Design review of the part built by this model. Coordinates are the model's own, in mm. A direction names the side the tool comes from. Round coordinates to 2 decimals unless told otherwise and drop trailing zeros. Loops run counter-clockwise (first coordinate to the right, second up) from the corner with the lowest first, then second, coordinate; pieces in that order, holes last. Notation, with made-up numbers: (24.5, -16) - (74.5, -16) arc R12 cw to (74.5, -1) - close; hole circle Ø3 at (-23.5, 29.5). An arc over 180 degrees is marked (long way). Return JSON: item names as keys, results as strings. Group by question number.
(1) For faces 1 (the flat face through (-35, 14, -54)), 2 (the cylindrical face through (-37.028, 16.354, -4.888)), 3 (the flat face through (-39, 13, -54)), list the 3-axis set-ups (+Z, -Z, +X, -X, +Y, -Y) from which the entire face can be reached by the end or side of a thin tool; tool diameter is ignored.
(2) The part is to be moulded in two halves that separate along X. For faces 4 (the cylindrical face through (-37.03, 17.69, -51.32)), 5 (the cylindrical face through (-42.33, 1.97, -51.95)), 6 (the flat face through (-35, 14, -5)), say which applies: pulls with the +X half, pulls with the -X half, needs draft (parallel to the pull), parting line crosses it, or undercut.
(3) We need section A-A, the plane x = -36.5. Write out the cut boundary in (y, z), and give its area (3 significant figures).
(4) Clearance check with flat-ended pins moving along their axes: pin 1 (4 mm diameter, centred on x = -32.5, z = -21.5, fed in from +Y); pin 2 (3 mm diameter, centred on x = -37, z = -51.5, fed in from +Y); pin 3 (2.5 mm diameter, centred on y = 14, z = -55, fed in from -X). State where each tip first meets the part, or that it passes through.
(5) We need section C-C, the plane z = -18.45. Write out the cut boundary in (x, y).
(6) We need section D-D, the plane z = -53.4. Write out the cut boundary in (x, y), and give its area (3 significant figures).
(7) We need section B-B, the plane y = 8.55. Write out the cut boundary in (x, z), and give its area (3 significant figures).
(8) Wall thickness on L1, parallel to Z at x = -37.5, y = 18.75; L2, parallel to Y at x = -37.65, z = -4.4; L3, parallel to X at y = 5.75, z = -2.5: over which ranges is each line inside the solid? List them lowest first. Write a range as [from, to].
from build123d import *

# Parameters (mm, degrees)
BOSS_EXTRUDE1_DEPTH = 4
SKETCH2_W           = 8.95
SKETCH2_H           = 19
SKETCH2_R           = 2.25
BOSS_EXTRUDE2_DEPTH = 4
FILLET1_R           = 10
FILLET2_R           = 4
SKETCH3_W           = 58.4
SKETCH3_H           = 19.3
SKETCH3_R           = 2
BOSS_EXTRUDE3_DEPTH = 4
FILLET3_R           = 10


with BuildPart() as part:
    # Sketch1 → Boss-Extrude1 (new body)
    with BuildSketch(Plane(origin=(0, 0, 0), x_dir=(1, 0, 0), z_dir=(0, 1, 0))):
        Polygon((-49, 49.45), (-39, 49.45), (-39, 58.4), (0, 58.4), (0, 0), (-39, 0), (-39, 8.95), (-49, 8.95), align=None)
    extrude(amount=BOSS_EXTRUDE1_DEPTH)

    # Sketch2 → Boss-Extrude2 (add)
    # profile 1 of 2: a face of its own
    with BuildSketch(Plane.ZY.offset(39)):
        with Locations((-4.475, 13.5)):
            Rectangle(SKETCH2_W, SKETCH2_H)
        with Locations((-4.4, 18.55)):
            Circle(SKETCH2_R, mode=Mode.SUBTRACT)
        with Locations((-4.4, 8.55)):
            Circle(SKETCH2_R, mode=Mode.SUBTRACT)
    # profile 2 of 2: a face of its own
    with BuildSketch(Plane.ZY.offset(39)):
        with Locations((-53.925, 13.5)):
            Rectangle(SKETCH2_W, SKETCH2_H)
        with Locations((-53.4, 18.55)):
            Circle(SKETCH2_R, mode=Mode.SUBTRACT)
        with Locations((-53.4, 8.55)):
            Circle(SKETCH2_R, mode=Mode.SUBTRACT)
    extrude(amount=-BOSS_EXTRUDE2_DEPTH)

    # Fillet1
    # the kernel refuses this fillet: 10 mm, written as the material it adds along each edge
    with BuildSketch(Plane(origin=(-39, 0, -49.45), x_dir=(-1, 0, 0), z_dir=(0, 1, 0))) as fillet1_piece_1:
        with BuildLine():
            CenterArc((9.944722218, -10), FILLET1_R, 90, 83.97283344)
            Line((0, -8.95), (0, 0))
            Line((0, 0), (9.944722218, 0))
        make_face()
    extrude(amount=4)
    with BuildSketch(Plane(origin=(-39, 0, -8.95), x_dir=(0, 0, 1), z_dir=(0, 1, 0))) as fillet1_piece_2:
        with BuildLine():
            CenterArc((10, -9.944722218), FILLET1_R, 96.02716656, 83.97283344)
            Line((0, -9.944722218), (0, 0))
            Line((0, 0), (8.95, 0))
        make_face()
    extrude(amount=4)

    # Fillet2
    fillet2_edges = [part.edges().sort_by_distance(p)[0] for p in [
        (-37, 23, 0),
        (-37, 23, -58.4),
    ]]
    fillet(fillet2_edges, radius=FILLET2_R)

    # Sketch3 → Boss-Extrude3 (add)
    with BuildSketch(Plane(origin=(0, 0, 0), x_dir=(0, 0, -1), z_dir=(1, 0, 0))):
        with Locations((29.2, 13.65)):
            Rectangle(SKETCH3_W, SKETCH3_H)
        with Locations((18.45, 13.55)):
            Circle(SKETCH3_R, mode=Mode.SUBTRACT)
    extrude(amount=-BOSS_EXTRUDE3_DEPTH)

    # Fillet3
    fillet3_edges = [part.edges().sort_by_distance(p)[0] for p in [
        (-2, 23.3, 0),
        (-2, 23.3, -58.4),
    ]]
    fillet(fillet3_edges, radius=FILLET3_R)


solid = part.part
Solutions:
{
 "1": {"face 1": "+Z, -Z, +Y", "face 2": "-X", "face 3": "+Z, -Z, -X, +Y"},
 "2": {"face 4": "needs draft", "face 5": "pulls with the -X half", "face 6": "undercut"},
 "3": {"outline": "(0, -58.4) - (19, -58.4) arc R4 ccw to (23, -54.4) - (23, -49.45) - (4, -49.45) - (4, -8.95) - (23, -8.95) - (23, -4) arc R4 ccw to (19, 0) - (0, 0) - close; hole circle Ø4.5 at (8.55, -53.4); hole circle Ø4.5 at (8.55, -4.4); hole circle Ø4.5 at (18.55, -53.4); hole circle Ø4.5 at (18.55, -4.4)", "area": "503 mm^2"},
 "4": {"pin 1": "y = 4", "pin 2": "y = 23", "pin 3": "x = -39"},
 "5": {"outline": "(-49, 0) - (0, 0) - (0, 11.55) - (-4, 11.55) - (-4, 4) - (-49, 4) - close; (-4, 15.55) - (0, 15.55) - (0, 23.3) - (-4, 23.3) - close"},
 "6": {"outline": "(-40.98, 0) - (0, 0) - (0, 21.96) - (-4, 21.96) - (-4, 4) - (-35, 4) - (-35, 6.3) - (-39, 6.3) - (-39, 4) - (-40.98, 4) - close; (-39, 10.8) - (-35, 10.8) - (-35, 16.3) - (-39, 16.3) - close; (-39, 20.8) - (-35, 20.8) - (-35, 23) - (-39, 23) - close", "area": "276 mm^2"},
 "7": {"outline": "(-39, -58.4) - (-35, -58.4) - (-35, -55.65) - (-39, -55.65) - close; (-39, -51.15) - (-35, -51.15) - (-35, -49.45) - (-39, -49.45) - close; (-39, -8.95) - (-35, -8.95) - (-35, -6.65) - (-39, -6.65) - close; (-39, -2.15) - (-35, -2.15) - (-35, 0) - (-39, 0) - close; (-4, -58.4) - (0, -58.4) - (0, 0) - (-4, 0) - close", "area": "269 mm^2"},
 "8": {"L1": "[-58.4, -55.64], [-51.16, -49.45], [-8.95, -6.64], [-2.16, 0]", "L2": "[0, 6.3], [10.8, 16.3], [20.8, 23]", "L3": "[-39, -35], [-4, 0]"}
}
